Here's how the part is built. I have some questions about the finished solid (model axes, mm). Face numbers are marked on the shaded views. A direction names the side the tool comes from. Coordinates: 2 decimals unless noted, no trailing zeros. Write each loop counter-clockwise with the first axis right and the second up, starting at its lowest first coordinate (ties: lowest second). Pieces come first, ordered by that corner, then holes.
(1) Which directions (+Z, -Z, +X, -X, +Y, -Y) give clear straight access to the entire face, cutting with the end or side of a thin tool? Please do the marked faces 1, 2 and 3.
(2) Imagine slicing it at C-C, the plane x = 8.5. List the corners of the cut face in (y, z) for me.
(3) Imagine slicing it at A-A, the plane y = 0. List the corners of the cut face in (x, z) for me, plus the area to 3 significant figures.
(4) For pin 1 Ø6 at (x, y) = (4, -10) entering from -Z; pin 2 Ø5 at (x, z) = (6, 27) entering from +Y; pin 3 Ø1.5 at (x, y) = (7, 21.5) entering from -Z, each with a flat end and sliding along its axis, tell me the tip position at first contact or that it passes through.
(5) Imagine slicing it at D-D, the plane z = 9. List the corners of the cut face in (x, y) for me, plus the area to 3 significant figures.
(6) Imagine slicing it at B-B, the plane z = -3.5. List the corners of the cut face in (x, y) for me, plus the area to 3 significant figures.
(7) Please list where these lines run through material, in increasing order: probe 1 along Z at (x, y) = (2.5, 0); probe 2 along Z at (x, y) = (8.25, -3.5); probe 3 along Y at (x, z) = (6.75, -11).
(8) Thinking about a two-plate mould opening in Y: for the marked faces 4, 5 and 6, which applies, released by +Y, released by -Y, zero draft, split by the parting line, or undercut?
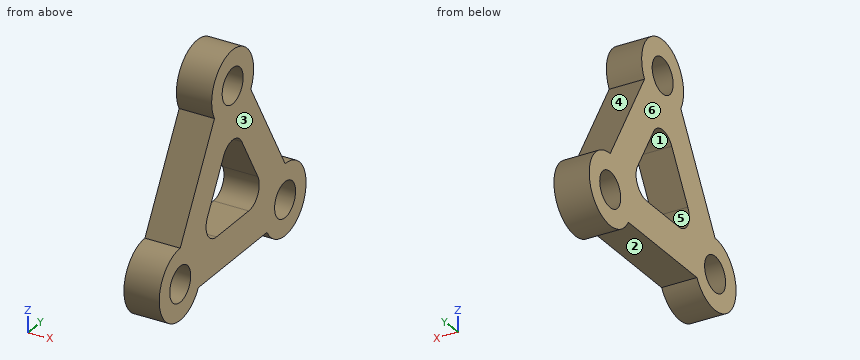
```python
from build123d import *

# Parameters (mm, degrees)
F0_R     = 5
F1_DEPTH = 10


with BuildPart() as f1:
    # F0 (on Right) → F1 (new body)
    with BuildSketch(Plane.YZ):
        with BuildLine():
            Line((25.000001, -4.433757), (8.660254, 23.867514))
            ThreePointArc((8.660254, 23.867514), (0, 38.867513), (-8.660254, 23.867513))
            Line((-8.660254, 23.867513), (-25, -4.433757))
            ThreePointArc((-25, -4.433757), (-33.660254, -19.433756), (-16.339746, -19.433757))
            Line((-16.339746, -19.433757), (16.339746, -19.433757))
            ThreePointArc((16.339746, -19.433757), (33.660254, -19.433757), (25.000001, -4.433757))
        make_face()
        with Locations((-25, -14.433757)):
            Circle(F0_R, mode=Mode.SUBTRACT)
        with Locations((25, -14.433757)):
            Circle(F0_R, mode=Mode.SUBTRACT)
        with BuildLine():
            ThreePointArc((-4.330127, 11.367513), (0, 13.867513), (4.330127, 11.367513))
            Line((4.330127, 11.367513), (12.009619, -1.933757))
            ThreePointArc((12.009619, -1.933757), (12.009619, -6.933757), (7.679492, -9.433757))
            Line((7.679492, -9.433757), (-7.679492, -9.433757))
            ThreePointArc((-7.679492, -9.433757), (-12.009619, -6.933757), (-12.009619, -1.933757))
            Line((-12.009619, -1.933757), (-4.330127, 11.367513))
        make_face(mode=Mode.SUBTRACT)
        with Locations((0, 28.867513)):
            Circle(F0_R, mode=Mode.SUBTRACT)
    extrude(amount=F1_DEPTH)


solid = f1.part
```
Recorded:
1. face 1: +X, -X
1. face 2: -Z, +X, -X
1. face 3: +Z, -Z, +X, +Y, -Y
2. outline: (-25, -4.43) arc R10 ccw (long way) to (-16.34, -19.43) - (16.34, -19.43) arc R10 ccw (long way) to (25, -4.43) - (8.66, 23.87) arc R10 ccw (long way) to (-8.66, 23.87) - close; hole circle Ø10 at (-25, -14.43); hole (-12.01, -1.93) arc R5 ccw to (-7.68, -9.43) - (7.68, -9.43) arc R5 ccw to (12.01, -1.93) - (4.33, 11.37) arc R5 ccw to (-4.33, 11.37) - close; hole circle Ø10 at (0, 28.87); hole circle Ø10 at (25, -14.43)
3. outline: (0, -19.43) - (10, -19.43) - (10, -9.43) - (0, -9.43) - close; (0, 13.87) - (10, 13.87) - (10, 23.87) - (0, 23.87) - close; (0, 33.87) - (10, 33.87) - (10, 38.87) - (0, 38.87) - close
3. area: 250 mm2
4. pin 1: stops at z = -19.43
4. pin 2: stops at y = 10
4. pin 3: stops at z = -24.05
5. outline: (0, -17.24) - (10, -17.24) - (10, -5.7) - (0, -5.7) - close; (0, 5.7) - (10, 5.7) - (10, 17.24) - (0, 17.24) - close
5. area: 231 mm2
6. outline: (0, -24.46) - (10, -24.46) - (10, -12.59) - (0, -12.59) - close; (0, 12.59) - (10, 12.59) - (10, 24.46) - (0, 24.46) - close
6. area: 237 mm2
7. probe 1: z = -19.43 to -9.43, 13.87 to 23.87, 33.87 to 38.87
7. probe 2: z = -19.43 to -9.43, 12.44 to 25.3, 32.44 to 38.24
7. probe 3: y = -34.39 to -28.63, -21.37 to 21.37, 28.63 to 34.39
8. face 4: released by +Y
8. face 5: undercut
8. face 6: zero draft
